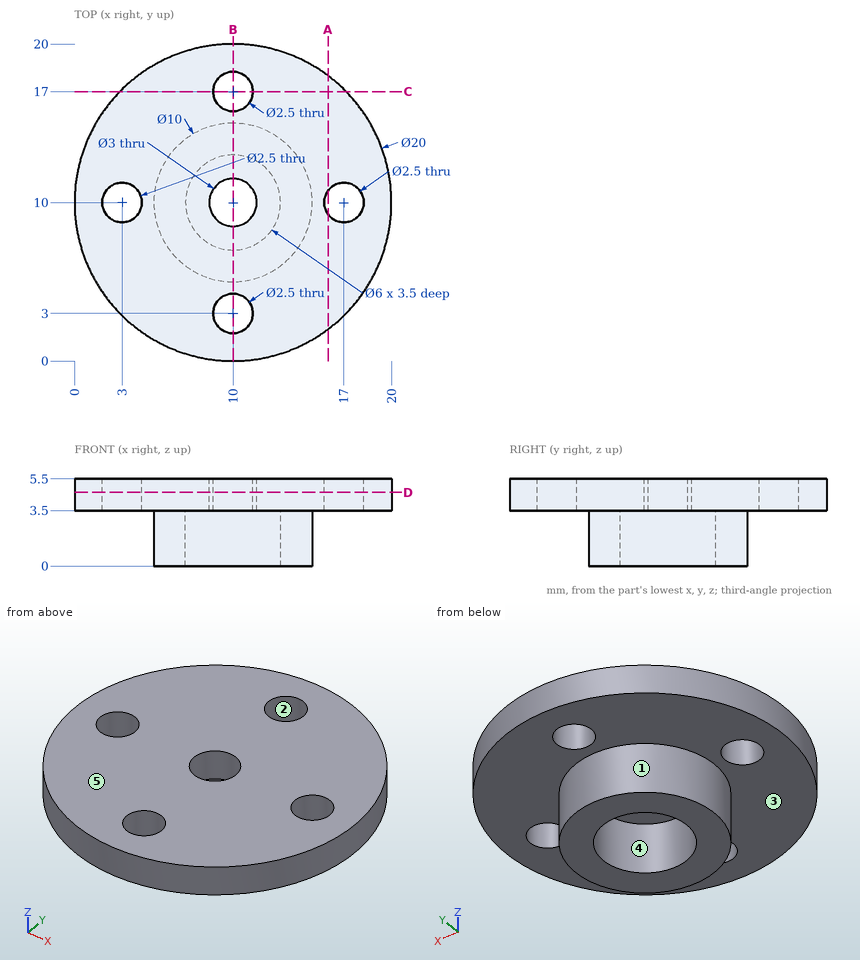
Here's the drawing with two shaded views (mm, measured from the low corner). I have some questions. A direction names the side the tool comes from. Give positions to 0.01 mm unless a question says otherwise; leave off trailing zeros. Loops run counter-clockwise (first coordinate to the right, second up) from the corner with the lowest first, then second, coordinate; pieces in that order, holes last. Notation, with made-up numbers: M -11.75,48 L 36.25,48 A27 ccw 36.25,71 Z; hole C 1,70 d2. An arc over 180 degrees is marked long. One line per item, written item: value. Start each with the question number.
1) If we section it at A-A, the plane x = 16: Write out the boundary of the cut face in (y, z), and give its area (3 significant figures).
2) On a 3-axis mill with a long thin cutter (end or side, diameter ignored), from which of +Z, -Z, +X, -X, +Y, -Y can I reach the whole of each face in a straight line? I mean the marked faces 4 and 5. Say none if no direction works.
3) Thinking about a two-plate mould opening in Y: for the marked faces 1, 2 and 3, which applies, +Y half, -Y half, draft (parallel to the pull), parting line (faces both ways), or undercut?
4) If we section it at D-D, the plane z = 4.65: Write out the boundary of the cut face in (x, y).
5) If we section it at B-B, the plane x = 10: Write out the boundary of the cut face in (y, z).
6) I'm going to push flat-ended pins straight in: pin 1 (2 mm diameter, centred on x = 3.5, y = 14.5, fed in from -Z); pin 2 (2 mm diameter, centred on y = 13.5, z = 1, fed in from -X); pin 3 (1.5 mm diameter, centred on x = 10, y = 17, fed in from -Z). Where does each tip first touch, or does it pass through?
7) If we section it at C-C, the plane y = 17: Write out the boundary of the cut face in (x, z).
8) If I drill on line 1 (X direction, y = 10, z = 4.65); line 2 (X direction, y = 10, z = 0.75), over which ranges is the centre line in solid material (lowest first)? Write a range as [from, to].
Completed:
1. outline: M 2,3.5 L 9.25,3.5 L 9.25,5.5 L 2,5.5 Z; M 10.75,3.5 L 18,3.5 L 18,5.5 L 10.75,5.5 Z
1. area: 29.0 mm^2
2. face 4: -Z
2. face 5: +Z, +X, -X, +Y, -Y
3. face 1: parting line
3. face 2: undercut
3. face 3: draft
4. outline: C 10,10 d20; hole C 3,10 d2.5; hole C 10,10 d3; hole C 10,3 d2.5; hole C 10,17 d2.5; hole C 17,10 d2.5
5. outline: M 0,3.5 L 1.75,3.5 L 1.75,5.5 L 0,5.5 Z; M 4.25,3.5 L 5,3.5 L 5,0 L 7,0 L 7,3.5 L 8.5,3.5 L 8.5,5.5 L 4.25,5.5 Z; M 11.5,3.5 L 13,3.5 L 13,0 L 15,0 L 15,3.5 L 15.75,3.5 L 15.75,5.5 L 11.5,5.5 Z; M 18.25,3.5 L 20,3.5 L 20,5.5 L 18.25,5.5 Z
6. pin 1: stops at z = 3.5
6. pin 2: stops at x = 5.67
6. pin 3: passes through
7. outline: M 2.86,3.5 L 8.75,3.5 L 8.75,5.5 L 2.86,5.5 Z; M 11.25,3.5 L 17.14,3.5 L 17.14,5.5 L 11.25,5.5 Z
8. line 1: x = [0, 1.75], [4.25, 8.5], [11.5, 15.75], [18.25, 20]
8. line 2: x = [5, 7], [13, 15]
